Answer from the drawing. Dimensions are ordinates in mm from the lowest x, y and z of the part. Round coordinates to 2 decimals unless told otherwise and drop trailing zeros. Write each loop counter-clockwise with the first axis right and the second up, starting at its lowest first coordinate (ties: lowest second). Pieces come first, ordered by that corner, then holes. Notation, with made-up numbers: (75.5, 42.25) -> (87.5, 42.25) arc R19 cw to (87.5, 67.25) -> close; hole circle Ø1 at (-33, 27.25). An arc over 180 degrees is marked (long way). Answer as a JSON object with one key per item and string values. Group by question number.
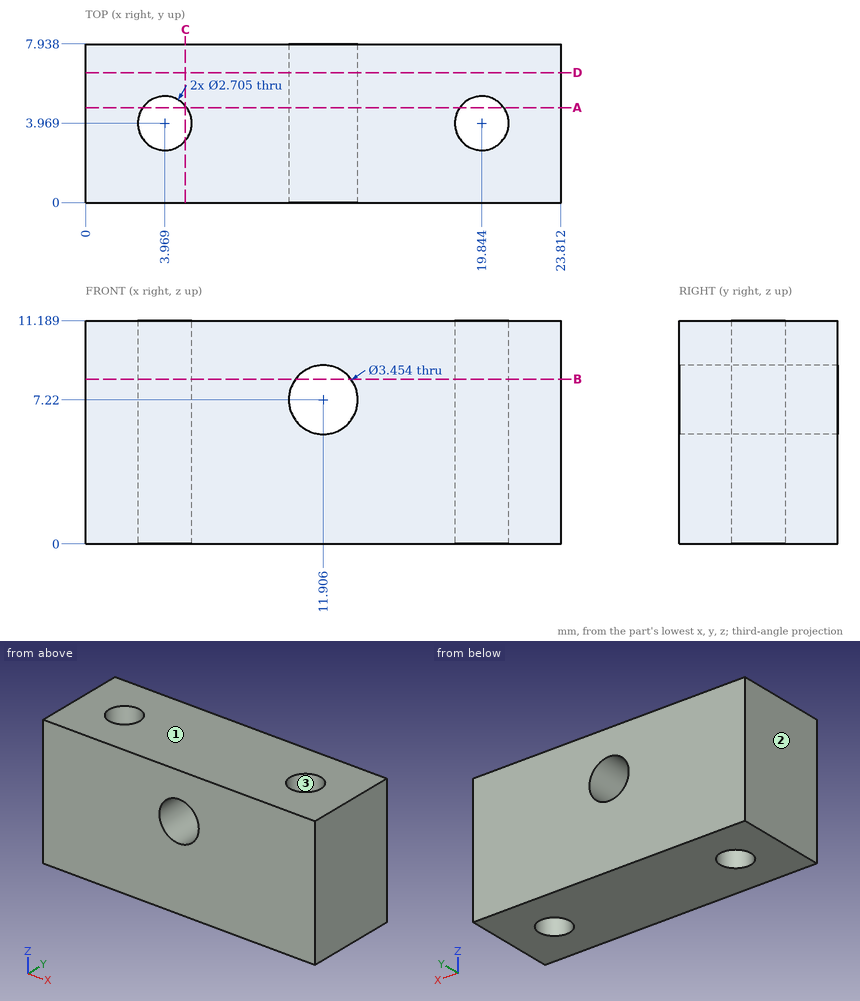
1) A cutting plane is placed at D-D on y = 6.5. Determine the outline of the cut face in (x, z) (1 decimal).
2) For a pull along X with two mould halves and no side action, classify the marked faces 1, 2 and 3 as released by +X, released by -X, zero draft, split by the parting line, or undercut.
3) This flat-tipped pin is pushed along its axis until it touches: P1, Ø4, axis at x = 12, z = 7, coming from the +Y side. Where does it stop, or does it pass through?
4) A cutting plane is placed at C-C on x = 5. Determine the outline of the cut face in (y, z).
5) A cutting plane is placed at A-A on y = 4.75. Determine the outline of the cut face in (x, z) (1 decimal), plus the area to 3 significant figures.
6) A cutting plane is placed at B-B on z = 8.25. Determine the outline of the cut face in (x, y) (1 decimal).
7) Straight lines are drawn through the part: L1, parallel to X at y = 4, z = 1 (1 decimal); L2, parallel to X at y = 4.5, z = 8.75 (1 decimal); L3, parallel to X at y = 5, z = 2 (1 decimal). For each, find the intervals that lie inside material, in ascending order.
Established:
{
 "1": {"outline": "(0, 0) -> (23.8, 0) -> (23.8, 11.2) -> (0, 11.2) -> close; hole circle Ø3.5 at (11.9, 7.2)"},
 "2": {"face 1": "zero draft", "face 2": "released by -X", "face 3": "undercut"},
 "3": {"P1": "stops at y = 7.94"},
 "4": {"outline": "(0, 0) -> (3.09, 0) -> (3.09, 11.19) -> (0, 11.19) -> close; (4.84, 0) -> (7.94, 0) -> (7.94, 11.19) -> (4.84, 11.19) -> close"},
 "5": {"outline": "(0, 0) -> (2.9, 0) -> (2.9, 11.2) -> (0, 11.2) -> close; (5.1, 0) -> (18.7, 0) -> (18.7, 11.2) -> (5.1, 11.2) -> close; (20.9, 0) -> (23.8, 0) -> (23.8, 11.2) -> (20.9, 11.2) -> close; hole circle Ø3.5 at (11.9, 7.2)", "area": "208 mm²"},
 "6": {"outline": "(0, 0) -> (10.5, 0) -> (10.5, 7.9) -> (0, 7.9) -> close; (13.3, 0) -> (23.8, 0) -> (23.8, 7.9) -> (13.3, 7.9) -> close; hole circle Ø2.7 at (4, 4); hole circle Ø2.7 at (19.8, 4)"},
 "7": {"L1": "x = 0 to 2.6, 5.3 to 18.5, 21.2 to 23.8", "L2": "x = 0 to 2.7, 5.2 to 11.1, 12.7 to 18.6, 21.1 to 23.8", "L3": "x = 0 to 3.1, 4.8 to 19, 20.7 to 23.8"}
}
